```python
from build123d import *

# Parameters (mm, degrees)
SKETCH151_R             = 4
SKETCH151_R_2           = 1.75
POCKET057_DEPTH         = 84.080664
POLARPATTERN010_COUNT   = 4
SKETCH176_W             = 20.848927
SKETCH176_H             = 11.039979
POCKET062_DEPTH         = 5.001
BODY104_PLACEMENT_ANGLE = 270


with BuildPart() as part:
    # Sketch150 → Revolution007 (revolve)
    with BuildSketch(Plane.YZ):
        Polygon((0, 0), (0, 15), (5.1, 15), (5.1, 13.5), (11, 13.5), (11, 10), (5.1, 10), (5.1, 0), align=None)
    revolve(axis=Axis((0, 0, 0), (0, 0, 1)))

    # Sketch151 (on Face1 of Revolution007) → Pocket057 (cut, through all)
    with BuildSketch(Plane(origin=(0, 0, 15), x_dir=(0, -1, 0), z_dir=(0, 0, 1))):
        Circle(SKETCH151_R)
        with Locations((8, 0)):
            Circle(SKETCH151_R_2)
    pocket057 = extrude(amount=-POCKET057_DEPTH, mode=Mode.SUBTRACT)

    # PolarPattern010: Pocket057 ×4 about axis
    polarpattern010_axis = Axis((0, 0, 15), (0, 0, 1))
    for i in range(1, POLARPATTERN010_COUNT):
        add(pocket057.rotate(polarpattern010_axis, i * 360 / POLARPATTERN010_COUNT), mode=Mode.SUBTRACT)

    # Sketch176 (on Face9 of Clone047) → Pocket062 (cut, through all)
    with BuildSketch(Plane(origin=(0, 0, 10), x_dir=(1, 0, 0), z_dir=(0, 0, -1))):
        with Locations((-0.416263, -13.519989)):
            Rectangle(SKETCH176_W, SKETCH176_H)
    extrude(amount=-POCKET062_DEPTH, mode=Mode.SUBTRACT)


with BuildPart() as part_1:
    # Body104 placement: moved
    add(part.part.moved(Location((30.052038, 4.5, 5.760408))).rotate(Axis((30.052038, 4.5, 5.760408), (1, 0, 0)), BODY104_PLACEMENT_ANGLE))


solid = part_1.part
```
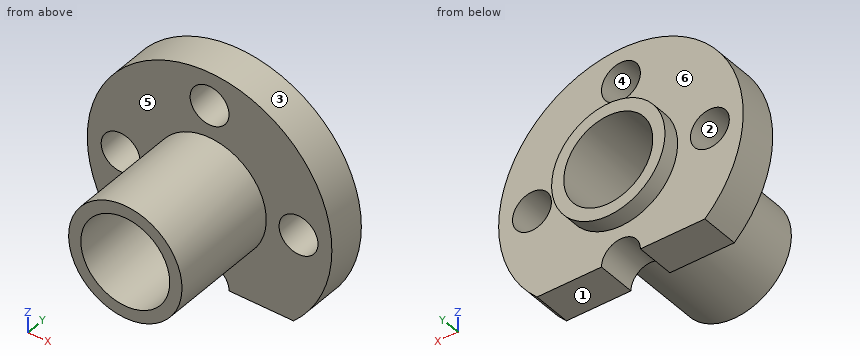
Read the model definition and answer for the solid it produces. Units are mm, in the model's axes. Face numbers are marked on the shaded views. A direction names the side the tool comes from. Coordinates: 2 decimals unless noted, no trailing zeros. Write each loop counter-clockwise with the first axis right and the second up, starting at its lowest first coordinate (ties: lowest second). Pieces come first, ordered by that corner, then holes. Notation, with made-up numbers: (-2, 66) -> (3, 66) arc R16 ccw to (3, 73) -> close; hole circle Ø5 at (8, -6). An arc over 180 degrees is marked (long way). Return JSON: item names as keys, results as strings.
1. Determine the mould class of the marked faces 1, 2 and 3 for opening direction Z: pulls with the +Z half, pulls with the -Z half, needs draft (parallel to the pull), parting line crosses it, or undercut.
Found:
{"face 1": "pulls with the -Z half", "face 2": "undercut", "face 3": "parting line crosses it"}
2. Each of these flat-tipped pins is pushed along its axis until it touches: P1, Ø1.5, axis at x = 35.5, y = 12.5, coming from the -Z side; P2, Ø3, axis at x = 34, y = 7.5, coming from the -Z side; P3, Ø5, axis at x = 27, z = 14, coming from the +Y side; P4, Ø1.5, axis at x = 28.5, y = 17.5, coming from the -Z side. Where does it stop, or does it pass through?
Found:
{"P1": "z = 3.78", "P2": "z = 1.29", "P3": "y = 18", "P4": "z = -2.24"}
3. A cutting plane is placed at C-C (y = 16.75). Determine the outline of the cut face in (x, z), and give its area (3 significant figures).
Found:
{"outline": "(22.5, -2.24) -> (28.3, -2.24) arc R1.75 cw to (31.8, -2.24) -> (37.6, -2.24) arc R11 ccw (long way) to start; hole circle Ø3.5 at (22.05, 5.76); hole circle Ø8 at (30.05, 5.76); hole circle Ø3.5 at (30.05, 13.76); hole circle Ø3.5 at (38.05, 5.76)", "area": "265 mm2"}
4. A cutting plane is placed at D-D (z = 6.5). Determine the outline of the cut face in (x, y).
Found:
{"outline": "(19.08, 14.5) -> (20.47, 14.5) -> (20.47, 18) -> (19.08, 18) -> close; (23.64, 14.5) -> (25.01, 14.5) -> (25.01, 4.5) -> (26.12, 4.5) -> (26.12, 19.5) -> (25.01, 19.5) -> (25.01, 18) -> (23.64, 18) -> close; (33.98, 4.5) -> (35.1, 4.5) -> (35.1, 14.5) -> (36.47, 14.5) -> (36.47, 18) -> (35.1, 18) -> (35.1, 19.5) -> (33.98, 19.5) -> close; (39.64, 14.5) -> (41.03, 14.5) -> (41.03, 18) -> (39.64, 18) -> close"}
5. A cutting plane is placed at B-B (z = 9.25). Determine the outline of the cut face in (x, y), and give its area (3 significant figures).
Found:
{"outline": "(19.62, 14.5) -> (26.33, 14.5) -> (26.33, 4.5) -> (28.1, 4.5) -> (28.1, 19.5) -> (26.33, 19.5) -> (26.33, 18) -> (19.62, 18) -> close; (32.01, 4.5) -> (33.77, 4.5) -> (33.77, 14.5) -> (40.48, 14.5) -> (40.48, 18) -> (33.77, 18) -> (33.77, 19.5) -> (32.01, 19.5) -> close", "area": "99.9 mm2"}
6. A cutting plane is placed at A-A (x = 31.5). Determine the outline of the cut face in (y, z), and give its area (3 significant figures).
Found:
{"outline": "(4.5, 0.87) -> (14.5, 0.87) -> (14.5, -1.26) -> (18, -1.26) -> (18, 0.87) -> (19.5, 0.87) -> (19.5, 2.03) -> (4.5, 2.03) -> close; (4.5, 9.49) -> (19.5, 9.49) -> (19.5, 10.65) -> (18, 10.65) -> (18, 12.78) -> (14.5, 12.78) -> (14.5, 10.65) -> (4.5, 10.65) -> close; (14.5, 14.74) -> (18, 14.74) -> (18, 16.66) -> (14.5, 16.66) -> close", "area": "56.5 mm2"}
7. Find the intervals of material crossed by line 1 along Z through (x, y) = (28.75, 17); line 2 along Y through (x, z) = (23.5, 1.25); line 3 along Z through (x, y) = (26.5, 5), in increasing order. Write a range as from..to.
Found:
{"line 1": "-1.07..1.98, 9.54..12.59, 14.93..16.68", "line 2": "14.5..18", "line 3": "2.1..3.92, 7.6..9.42"}
8. A tool of negligible diameter and unlimited length cuts with its end or side. For the marked faces 4, 5 and 6, from which of +Z, -Z, +X, -X, +Y, -Y can it reach the whole face along a straight path? Write none if from no direction.
Found:
{"face 4": "+Y, -Y", "face 5": "-Y", "face 6": "+Y"}
